Check sheet for the drawn part. Datum: minimum x, y, z corner. Units: mm. Coordinates: 2 decimals unless noted, no trailing zeros. Order: outer loops, then holes, each group sorted by start corner. A loop starts at its lowest first (then second) coordinate and runs counter-clockwise, first axis right, second up. Notation, with made-up numbers: (86.5, 48.25) - (127.5, 48.25) arc R29 cw to (127.5, 83.25) - close; hole circle Ø11 at (18.5, 57.25). An arc over 180 degrees is marked (long way). One line per item, written item: value. Start each with the question number.
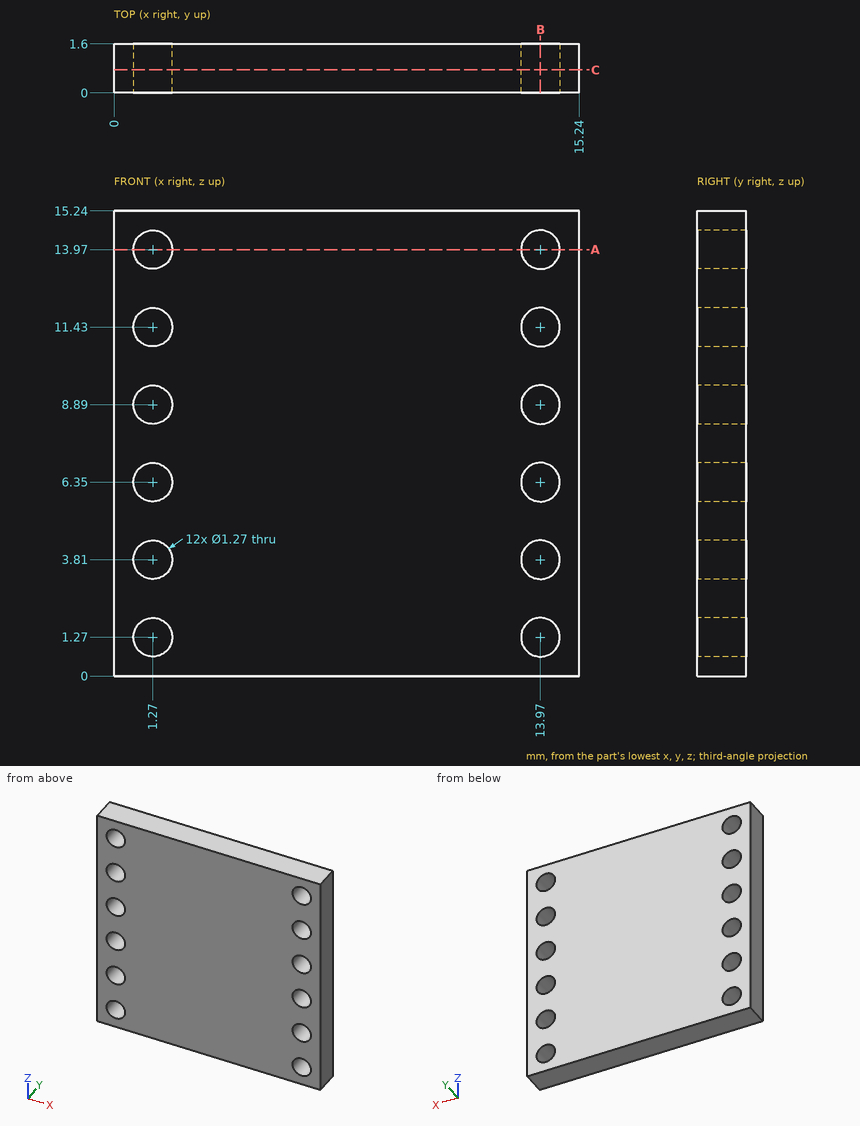
Q1. Material ranges on probe 1 along X at (y, z) = (0.65, 13.97) (3 decimals); probe 2 along X at (y, z) = (0.9, 8.75), recorded low to high.
Q2. Cross-section at B-B, the plane x = 13.97. Enter the section's corners in (y, z) (3 decimals).
Q3. Cross-section at C-C, the plane y = 0.75. Count the separate pieces of the cut face and the enclosed holes in it, and give its area (3 significant figures).
Q4. Cross-section at A-A, the plane z = 13.97. Enter the section's corners in (x, y) (3 decimals).
Q5. Gauge pin test, flat end, axial feed: P1, Ø1.1, axis at x = 1.27, z = 6.35, coming from the -Y side. Record the tip position at first contact, or that the pin passes through.
Check result:
1. probe 1: x = 0 to 0.635, 1.905 to 13.335, 14.605 to 15.24
1. probe 2: x = 0 to 0.65, 1.89 to 13.35, 14.59 to 15.24
2. outline: (0, 0) - (1.6, 0) - (1.6, 0.635) - (0, 0.635) - close; (0, 1.905) - (1.6, 1.905) - (1.6, 3.175) - (0, 3.175) - close; (0, 4.445) - (1.6, 4.445) - (1.6, 5.715) - (0, 5.715) - close; (0, 6.985) - (1.6, 6.985) - (1.6, 8.255) - (0, 8.255) - close; (0, 9.525) - (1.6, 9.525) - (1.6, 10.795) - (0, 10.795) - close; (0, 12.065) - (1.6, 12.065) - (1.6, 13.335) - (0, 13.335) - close; (0, 14.605) - (1.6, 14.605) - (1.6, 15.24) - (0, 15.24) - close
3. separate pieces: 1
3. enclosed holes: 12
3. area: 217 mm2
4. outline: (0, 0) - (0.635, 0) - (0.635, 1.6) - (0, 1.6) - close; (1.905, 0) - (13.335, 0) - (13.335, 1.6) - (1.905, 1.6) - close; (14.605, 0) - (15.24, 0) - (15.24, 1.6) - (14.605, 1.6) - close
5. P1: passes through
